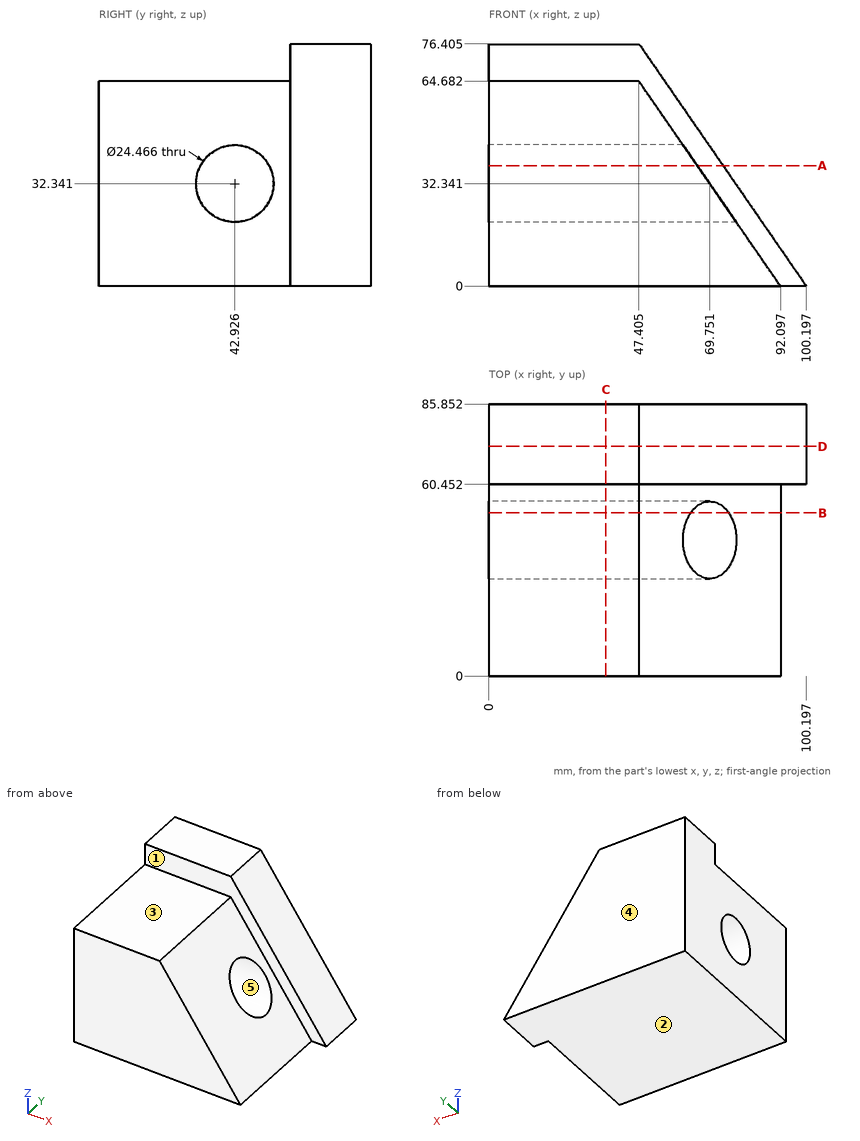
Geometry: see drawing. Coordinates: mm, zero at the bounding-box minimum. A direction names the side the tool comes from. Round coordinates to 2 decimals unless told otherwise and drop trailing zeros. Order: outer loops, then holes, each group sorted by start corner. A loop starts at its lowest first (then second) coordinate and runs counter-clockwise, first axis right, second up. Notation, with made-up numbers: (-38.5, 3) - (-32.5, 3) arc R5 ccw to (-32.5, 12) - close; hole circle Ø7 at (56.5, -26.75). An arc over 180 degrees is marked (long way). One line per question, with ' | ' between items. Start each with the question number.
1) Set-up query: the marked faces 1 and 2. Return all of +Z, -Z, +X, -X, +Y, -Y with unobstructed straight access to the full face (end or side cutting, diameter ignored); none if empty.
2) Cut plane D-D, the plane y = 72.5. Return the cut outline in (x, z) (1 decimal).
3) Pull-direction query (Z, two-part tool) for the marked faces 3, 4 and 5; classes: +Z half, -Z half, draft (parallel to the pull), parting line (faces both ways), or undercut.
4) Cut plane C-C, the plane x = 37. Return the cut outline in (y, z) (1 decimal), then the cut area to 3 significant figures.
5) Cut plane B-B, the plane y = 51.5. Return the cut outline in (x, z) (1 decimal).
6) Cut plane A-A, the plane z = 38. Return the cut outline in (x, y), then the cut area to 3 significant figures.
7) Contact query for flat-ended pins moving along their axis: P1, Ø10, axis at x = 46.5, z = 63, coming from the -Y side; P2, Ø14.5, axis at y = 42.93, z = 32.34, coming from the -X side; P3, Ø5, axis at x = 49.5, y = 22.5, coming from the +Z side; P4, Ø1, axis at x = 75, z = 28, coming from the -Y side. Output: stop coordinate, or through.
8) Ray query, probe 1 along Y at (x, z) = (21, 32.5); probe 2 along Z at (x, y) = (10.5, 26.5); probe 3 along Y at (x, z) = (44, 66.5). Return the intervals inside material, ascending.
Worked out:
1) face 1: +Z, +X, -Y | face 2: -Z, +X, -X, +Y, -Y
2) outline: (0, 0) - (100.2, 0) - (47.4, 76.4) - (0, 76.4) - close
3) face 3: +Z half | face 4: draft | face 5: undercut
4) outline: (0, 0) - (85.9, 0) - (85.9, 76.4) - (60.5, 76.4) - (60.5, 64.7) - (0, 64.7) - close; hole circle Ø24.5 at (42.9, 32.3) | area: 5,380 mm^2
5) outline: (0, 0) - (92.1, 0) - (75.8, 23.6) - (0, 23.6) - close; (0, 41.1) - (63.7, 41.1) - (47.4, 64.7) - (0, 64.7) - close
6) outline: (0, 0) - (65.84, 0) - (65.84, 32.08) - (0, 32.08) - close; (0, 53.77) - (65.84, 53.77) - (65.84, 60.45) - (73.94, 60.45) - (73.94, 85.85) - (0, 85.85) - close | area: 4,430 mm^2
7) P1: stops at y = 0 | P2: passes through | P3: stops at z = 64.68 | P4: stops at y = 60.45
8) probe 1: y = 0 to 30.69, 55.16 to 85.85 | probe 2: z = 0 to 64.68 | probe 3: y = 60.45 to 85.85
